from build123d import *

# Parameters (mm, degrees)
F0_R     = 4.1
F0_R_2   = 3
F1_DEPTH = 19
F3_DEPTH = 25


with BuildPart() as f1:
    # F0 (on Top) → F1 (new body)
    with BuildSketch(Plane.XY):
        Circle(F0_R)
        Circle(F0_R_2, mode=Mode.SUBTRACT)
        Circle(F0_R_2)
    extrude(amount=F1_DEPTH)

    # F2 (on face) → F3 (cut)
    with BuildSketch(Plane.XY.offset(19)):
        with BuildLine():
            ThreePointArc((0.4990696282, 4.0695121951), (0.4997673529, 4.0847490014), (0.5, 4.1))
            ThreePointArc((0.5, 4.1), (-0.0152509986, 4.5997673529), (-0.4990696282, 4.0695121951))
            ThreePointArc((-0.4990696282, 4.0695121951), (0, 4.1), (0.4990696282, 4.0695121951))
        make_face()
        with BuildLine():
            ThreePointArc((0.4990696282, 4.0695121951), (0, 4.1), (-0.4990696282, 4.0695121951))
            ThreePointArc((-0.4990696282, 4.0695121951), (0, 3.6), (0.4990696282, 4.0695121951))
        make_face()
        with BuildLine():
            ThreePointArc((-1.7321918491, 3.7161150948), (-1.2669696769, 3.8993317168), (-0.7829050052, 4.0245570878))
            ThreePointArc((-0.7829050052, 4.0245570878), (-1.4214781741, 4.374859975), (-1.7321918491, 3.7161150948))
        make_face()
        with BuildLine():
            ThreePointArc((-0.7669696769, 3.8993317168), (-0.7709695076, 3.9624493218), (-0.7829050052, 4.0245570878))
            ThreePointArc((-0.7829050052, 4.0245570878), (-1.2669696769, 3.8993317168), (-1.7321918491, 3.7161150948))
            ThreePointArc((-1.7321918491, 3.7161150948), (-1.1737256049, 3.4081031111), (-0.7669696769, 3.8993317168))
        make_face()
        with BuildLine():
            ThreePointArc((1.7321918491, 3.7161150948), (1.2669696769, 3.8993317168), (0.7829050052, 4.0245570878))
            ThreePointArc((0.7829050052, 4.0245570878), (1.1124611797, 3.4238034587), (1.7321918491, 3.7161150948))
        make_face()
        with BuildLine():
            ThreePointArc((-2.7957550629, 2.9989587574), (-2.4099195344, 3.3169696769), (-1.9882434418, 3.585650292))
            ThreePointArc((-1.9882434418, 3.585650292), (-2.7038121605, 3.7214781741), (-2.7957550629, 2.9989587574))
        make_face()
        with BuildLine():
            ThreePointArc((-1.9099195344, 3.3169696769), (-1.929899719, 3.4569017206), (-1.9882434418, 3.585650292))
            ThreePointArc((-1.9882434418, 3.585650292), (-2.4099195344, 3.3169696769), (-2.7957550629, 2.9989587574))
            ThreePointArc((-2.7957550629, 2.9989587574), (-2.2409783675, 2.8463754971), (-1.9099195344, 3.3169696769))
        make_face()
        with BuildLine():
            ThreePointArc((2.7957550629, 2.9989587574), (2.4099195344, 3.3169696769), (1.9882434418, 3.585650292))
            ThreePointArc((1.9882434418, 3.585650292), (2.1160269083, 2.9124611797), (2.7957550629, 2.9989587574))
        make_face()
        with BuildLine():
            ThreePointArc((-3.585650292, 1.9882434418), (-3.3169696769, 2.4099195344), (-2.9989587574, 2.7957550629))
            ThreePointArc((-2.9989587574, 2.7957550629), (-3.7214781741, 2.7038121605), (-3.585650292, 1.9882434418))
        make_face()
        with BuildLine():
            ThreePointArc((-2.8169696769, 2.4099195344), (-2.8647498964, 2.6232204254), (-2.9989587574, 2.7957550629))
            ThreePointArc((-2.9989587574, 2.7957550629), (-3.3169696769, 2.4099195344), (-3.585650292, 1.9882434418))
            ThreePointArc((-3.585650292, 1.9882434418), (-3.0764913073, 1.9715473709), (-2.8169696769, 2.4099195344))
        make_face()
        with BuildLine():
            ThreePointArc((3.585650292, 1.9882434418), (3.3169696769, 2.4099195344), (2.9989587574, 2.7957550629))
            ThreePointArc((2.9989587574, 2.7957550629), (2.9124611797, 2.1160269083), (3.585650292, 1.9882434418))
        make_face()
        with BuildLine():
            ThreePointArc((-4.0245570878, 0.7829050052), (-3.8993317168, 1.2669696769), (-3.7161150948, 1.7321918491))
            ThreePointArc((-3.7161150948, 1.7321918491), (-4.374859975, 1.4214781741), (-4.0245570878, 0.7829050052))
        make_face()
        with BuildLine():
            ThreePointArc((-3.3993317168, 1.2669696769), (-3.486047123, 1.5483872395), (-3.7161150948, 1.7321918491))
            ThreePointArc((-3.7161150948, 1.7321918491), (-3.8993317168, 1.2669696769), (-4.0245570878, 0.7829050052))
            ThreePointArc((-4.0245570878, 0.7829050052), (-3.5932375201, 0.8716137073), (-3.3993317168, 1.2669696769))
        make_face()
        with BuildLine():
            ThreePointArc((4.0245570878, 0.7829050052), (3.8993317168, 1.2669696769), (3.7161150948, 1.7321918491))
            ThreePointArc((3.7161150948, 1.7321918491), (3.4238034587, 1.1124611797), (4.0245570878, 0.7829050052))
        make_face()
        with BuildLine():
            ThreePointArc((-4.0695121951, -0.4990696282), (-4.1, 0), (-4.0695121951, 0.4990696282))
            ThreePointArc((-4.0695121951, 0.4990696282), (-4.6, 0), (-4.0695121951, -0.4990696282))
        make_face()
        with BuildLine():
            ThreePointArc((-3.6, 0), (-3.7358270312, 0.3426047997), (-4.0695121951, 0.4990696282))
            ThreePointArc((-4.0695121951, 0.4990696282), (-4.1, 0), (-4.0695121951, -0.4990696282))
            ThreePointArc((-4.0695121951, -0.4990696282), (-3.7358270312, -0.3426047997), (-3.6, 0))
        make_face()
        with BuildLine():
            ThreePointArc((4.1, 0), (4.0923709509, 0.25), (4.0695121951, 0.4990696282))
            ThreePointArc((4.0695121951, 0.4990696282), (3.6, 0), (4.0695121951, -0.4990696282))
            ThreePointArc((4.0695121951, -0.4990696282), (4.0923709509, -0.25), (4.1, 0))
        make_face()
        with BuildLine():
            ThreePointArc((4.6, 0), (4.4426047997, 0.3641729688), (4.0695121951, 0.4990696282))
            ThreePointArc((4.0695121951, 0.4990696282), (4.0923709509, 0.25), (4.1, 0))
            ThreePointArc((4.1, 0), (4.0923709509, -0.25), (4.0695121951, -0.4990696282))
            ThreePointArc((4.0695121951, -0.4990696282), (4.4426047997, -0.3641729688), (4.6, 0))
        make_face()
        with BuildLine():
            ThreePointArc((-3.7161150948, -1.7321918491), (-3.8993317168, -1.2669696769), (-4.0245570878, -0.7829050052))
            ThreePointArc((-4.0245570878, -0.7829050052), (-4.374859975, -1.4214781741), (-3.7161150948, -1.7321918491))
        make_face()
        with BuildLine():
            ThreePointArc((-3.3993317168, -1.2669696769), (-3.5932375201, -0.8716137073), (-4.0245570878, -0.7829050052))
            ThreePointArc((-4.0245570878, -0.7829050052), (-3.8993317168, -1.2669696769), (-3.7161150948, -1.7321918491))
            ThreePointArc((-3.7161150948, -1.7321918491), (-3.486047123, -1.5483872395), (-3.3993317168, -1.2669696769))
        make_face()
        with BuildLine():
            ThreePointArc((3.7161150948, -1.7321918491), (3.8993317168, -1.2669696769), (4.0245570878, -0.7829050052))
            ThreePointArc((4.0245570878, -0.7829050052), (3.4238034587, -1.1124611797), (3.7161150948, -1.7321918491))
        make_face()
        with BuildLine():
            ThreePointArc((-2.8169696769, -2.4099195344), (-3.0764913073, -1.9715473709), (-3.585650292, -1.9882434418))
            ThreePointArc((-3.585650292, -1.9882434418), (-3.3169696769, -2.4099195344), (-2.9989587574, -2.7957550629))
            ThreePointArc((-2.9989587574, -2.7957550629), (-2.8647498964, -2.6232204254), (-2.8169696769, -2.4099195344))
        make_face()
        with BuildLine():
            ThreePointArc((2.9989587574, -2.7957550629), (3.3169696769, -2.4099195344), (3.585650292, -1.9882434418))
            ThreePointArc((3.585650292, -1.9882434418), (2.9124611797, -2.1160269083), (2.9989587574, -2.7957550629))
        make_face()
        with BuildLine():
            ThreePointArc((-1.9099195344, -3.3169696769), (-2.2409783675, -2.8463754971), (-2.7957550629, -2.9989587574))
            ThreePointArc((-2.7957550629, -2.9989587574), (-2.4099195344, -3.3169696769), (-1.9882434418, -3.585650292))
            ThreePointArc((-1.9882434418, -3.585650292), (-1.929899719, -3.4569017206), (-1.9099195344, -3.3169696769))
        make_face()
        with BuildLine():
            ThreePointArc((1.9882434418, -3.585650292), (2.4099195344, -3.3169696769), (2.7957550629, -2.9989587574))
            ThreePointArc((2.7957550629, -2.9989587574), (2.1160269083, -2.9124611797), (1.9882434418, -3.585650292))
        make_face()
        with BuildLine():
            ThreePointArc((-0.7669696769, -3.8993317168), (-1.1737256049, -3.4081031111), (-1.7321918491, -3.7161150948))
            ThreePointArc((-1.7321918491, -3.7161150948), (-1.2669696769, -3.8993317168), (-0.7829050052, -4.0245570878))
            ThreePointArc((-0.7829050052, -4.0245570878), (-0.7709695076, -3.9624493218), (-0.7669696769, -3.8993317168))
        make_face()
        with BuildLine():
            ThreePointArc((0.7829050052, -4.0245570878), (1.2669696769, -3.8993317168), (1.7321918491, -3.7161150948))
            ThreePointArc((1.7321918491, -3.7161150948), (1.1124611797, -3.4238034587), (0.7829050052, -4.0245570878))
        make_face()
        with BuildLine():
            ThreePointArc((0.4990696282, -4.0695121951), (0, -3.6), (-0.4990696282, -4.0695121951))
            ThreePointArc((-0.4990696282, -4.0695121951), (0, -4.1), (0.4990696282, -4.0695121951))
        make_face()
    extrude(amount=-F3_DEPTH, mode=Mode.SUBTRACT)


solid = f1.part
Check sheet for the modelled part. Datum: model origin and axes. Units: mm. Coordinates: 2 decimals unless noted, no trailing zeros. Loops run counter-clockwise (first coordinate to the right, second up) from the corner with the lowest first, then second, coordinate; pieces in that order, holes last. Notation, with made-up numbers: (56, 43.5) -> (60, 43.5) arc R23 cw to (60, 53.5) -> close; hole circle Ø10 at (24.25, 42.5). An arc over 180 degrees is marked (long way). Write item = value, one per line. Start each with the question number.
1. Material ranges on line 1 (Y direction, x = 3.5, z = 12.5); line 2 (X direction, y = 3.25, z = 17.5); line 3 (X direction, y = 3.75, z = 2.25), recorded low to high.
2. Depth check by flat-ended pin: P1, Ø1.5, axis at x = -3, z = 11, coming from the -Y side. Enter the tip coordinate at first touch or a pass-through.
3. Draft check along Y on faces 1 (the cylindrical face through (0, -3.6, 9.6)), 2 (the cylindrical face through (3.43, -1.1, 9.63)), 3 (the flat face through (0, 0, 0)). Enter one of: released by +Y, released by -Y, zero draft, split by the parting line, or undercut.
4. Section check B-B on x = 1. Record the cut outline in (y, z), then the cut area to 3 significant figures.
5. Section check A-A on x = 0. Record the cut outline in (y, z).
Responses:
q1.line_1 = -1.94 to -1.57, -0.97 to 0.97, 1.57 to 1.94
q1.line_2 = -1.91 to 1.91
q1.line_3 = -0.79 to -0.36, 0.36 to 0.79
q2.P1 = -3
q3.face_1 = released by -Y
q3.face_2 = undercut
q3.face_3 = zero draft
q4.outline = (-3.48, 0) -> (3.48, 0) -> (3.48, 19) -> (-3.48, 19) -> close
q4.area = 132 mm2
q5.outline = (-3.6, 0) -> (3.6, 0) -> (3.6, 19) -> (-3.6, 19) -> close
